```python
from build123d import *

# Parameters (mm, degrees)
SKETCH_1_R          = 1.1
EXTRUDE_1_DEPTH     = 3
SKETCH_2_R          = 1.6
CUT_EXTRUDE_1_DEPTH = 137.736973785
SKETCH_5_R          = 1.35
CUT_EXTRUDE_3_DEPTH = 137.736973785
FILLET_1_R          = 5


with BuildPart() as part:
    # 草图1 → 凸台-拉伸1 (new body)
    with BuildSketch(Plane(origin=(0, 0, 0), x_dir=(1, 0, 0), z_dir=(0, 1, 0))):
        Polygon((0, 0), (128, 0), (128, 48), (110, 48), (18, 48), (0, 48), align=None)
        with Locations(Location((125, 8.5, 0), (0, 0, 270))):
            Circle(SKETCH_1_R, mode=Mode.SUBTRACT)
        with Locations(Location((113, 8.5, 0), (0, 0, 270))):
            Circle(SKETCH_1_R, mode=Mode.SUBTRACT)
        with Locations(Location((125, 16.5, 0), (0, 0, 270))):
            Circle(SKETCH_1_R, mode=Mode.SUBTRACT)
        with Locations(Location((113, 16.5, 0), (0, 0, 270))):
            Circle(SKETCH_1_R, mode=Mode.SUBTRACT)
        with Locations(Location((125, 31.5, 0), (0, 0, 90))):
            Circle(SKETCH_1_R, mode=Mode.SUBTRACT)
        with Locations(Location((125, 39.5, 0), (0, 0, 90))):
            Circle(SKETCH_1_R, mode=Mode.SUBTRACT)
        with Locations(Location((113, 39.5, 0), (0, 0, 90))):
            Circle(SKETCH_1_R, mode=Mode.SUBTRACT)
        with Locations(Location((113, 31.5, 0), (0, 0, 90))):
            Circle(SKETCH_1_R, mode=Mode.SUBTRACT)
        with Locations(Location((15, 8.5, 0), (0, 0, 90))):
            Circle(SKETCH_1_R, mode=Mode.SUBTRACT)
        with Locations(Location((3, 8.5, 0), (0, 0, 90))):
            Circle(SKETCH_1_R, mode=Mode.SUBTRACT)
        with Locations(Location((3, 16.5, 0), (0, 0, 90))):
            Circle(SKETCH_1_R, mode=Mode.SUBTRACT)
        with Locations(Location((15, 16.5, 0), (0, 0, 90))):
            Circle(SKETCH_1_R, mode=Mode.SUBTRACT)
        with Locations(Location((15, 39.5, 0), (0, 0, 270))):
            Circle(SKETCH_1_R, mode=Mode.SUBTRACT)
        with Locations(Location((3, 39.5, 0), (0, 0, 270))):
            Circle(SKETCH_1_R, mode=Mode.SUBTRACT)
        with Locations(Location((3, 31.5, 0), (0, 0, 270))):
            Circle(SKETCH_1_R, mode=Mode.SUBTRACT)
        with Locations(Location((15, 31.5, 0), (0, 0, 270))):
            Circle(SKETCH_1_R, mode=Mode.SUBTRACT)
    extrude(amount=EXTRUDE_1_DEPTH)

    # 草图2 → 切除-拉伸1 (cut, through all)
    with BuildSketch(Plane(origin=(0, 3, 0), x_dir=(1, 0, 0), z_dir=(0, 1, 0))):
        with Locations(Location((21.5, 20, 0), (0, 0, 270))):
            Circle(SKETCH_2_R)
        with Locations(Location((35.5, 20, 0), (0, 0, 270))):
            Circle(SKETCH_2_R)
        with Locations(Location((35.5, 6, 0), (0, 0, 270))):
            Circle(SKETCH_2_R)
        with Locations(Location((21.5, 6, 0), (0, 0, 270))):
            Circle(SKETCH_2_R)
        with Locations(Location((106.5, 6, 0), (0, 0, 90))):
            Circle(SKETCH_2_R)
        with Locations(Location((92.5, 6, 0), (0, 0, 90))):
            Circle(SKETCH_2_R)
        with Locations(Location((92.5, 20, 0), (0, 0, 90))):
            Circle(SKETCH_2_R)
        with Locations(Location((106.5, 20, 0), (0, 0, 90))):
            Circle(SKETCH_2_R)
    extrude(amount=-CUT_EXTRUDE_1_DEPTH, mode=Mode.SUBTRACT)

    # 草图5 → 切除-拉伸3 (cut, through all)
    with BuildSketch(Plane(origin=(0, 3, 0), x_dir=(1, 0, 0), z_dir=(0, 1, 0))):
        with Locations(Location((53.5, 42, 0), (0, 0, 270))):
            Circle(SKETCH_5_R)
        with Locations(Location((74.5, 42, 0), (0, 0, 90))):
            Circle(SKETCH_5_R)
        with Locations(Location((74.5, 30, 0), (0, 0, 270))):
            Circle(SKETCH_5_R)
        with Locations(Location((53.5, 30, 0), (0, 0, 90))):
            Circle(SKETCH_5_R)
    extrude(amount=-CUT_EXTRUDE_3_DEPTH, mode=Mode.SUBTRACT)

    # 圆角1
    fillet_1_edges = [part.edges().sort_by_distance(p)[0] for p in [
        (0, 1.5, -48),
        (128, 1.5, -48),
        (128, 1.5, 0),
        (0, 1.5, 0),
    ]]
    fillet(fillet_1_edges, radius=FILLET_1_R)


solid = part.part
```
Geometry: final body of the model. Coordinates: model frame, mm. Round coordinates to 2 decimals unless told otherwise and drop trailing zeros. Loops run counter-clockwise (first coordinate to the right, second up) from the corner with the lowest first, then second, coordinate; pieces in that order, holes last. Notation, with made-up numbers: (-13.75, 41.5) -> (18.25, 41.5) arc R37 ccw to (18.25, 79.5) -> close; hole circle Ø4 at (29.25, 65). An arc over 180 degrees is marked (long way). Use one line per item in the form item = value. Start each with the question number.
1) Section B-B on z = -16.5. Output: boundary loops of the cut face in (x, y).
2) Section A-A on x = 92.5. Output: boundary loops of the cut face in (y, z), then the cut area to 3 significant figures.
3) First-contact query: P1, Ø3.5, axis at x = 125, z = -31.5, coming from the -Y side. Flat tip, straight axial feed; report the tip coordinate or a pass-through.
4) Section C-C on y = 0.45. Give the number of separate pieces and of enclosed holes in the cut face, then the cut area to 3 significant figures.
5) Draft query along Z for faces 1 (the cylindrical face through (1, 2, -46)), 2 (the flat face through (63, 3, -24)), 3 (the cylindrical face through (3, 1.5, -15.4)). Return one class per face: released by +Z, released by -Z, zero draft, split by the parting line, or undercut.
6) Line query: L1, parallel to X at y = 1.7, z = -42; L2, parallel to X at y = 0.75, z = -39.5; L3, parallel to Z at x = 113, y = 0.7. Output: solid intervals per line, ascending.
Response:
q1.outline = (0, 0) -> (1.9, 0) -> (1.9, 3) -> (0, 3) -> close; (4.1, 0) -> (13.9, 0) -> (13.9, 3) -> (4.1, 3) -> close; (16.1, 0) -> (111.9, 0) -> (111.9, 3) -> (16.1, 3) -> close; (114.1, 0) -> (123.9, 0) -> (123.9, 3) -> (114.1, 3) -> close; (126.1, 0) -> (128, 0) -> (128, 3) -> (126.1, 3) -> close
q2.outline = (0, -48) -> (3, -48) -> (3, -21.6) -> (0, -21.6) -> close; (0, -18.4) -> (3, -18.4) -> (3, -7.6) -> (0, -7.6) -> close; (0, -4.4) -> (3, -4.4) -> (3, 0) -> (0, 0) -> close
q2.area = 125 mm^2
q3.P1 = 0
q4.separate_pieces = 1
q4.enclosed_holes = 28
q4.area = 5,970 mm^2
q5.face_1 = released by -Z
q5.face_2 = zero draft
q5.face_3 = undercut
q6.L1 = 0 to 52.15, 54.85 to 73.15, 75.85 to 128
q6.L2 = 0 to 1.9, 4.1 to 13.9, 16.1 to 111.9, 114.1 to 123.9, 126.1 to 128
q6.L3 = -48 to -40.6, -38.4 to -32.6, -30.4 to -17.6, -15.4 to -9.6, -7.4 to 0
